Input: part model. Units: mm. Frame: model coordinates. A direction names the side the tool comes from. Round coordinates to 2 decimals unless told otherwise and drop trailing zeros. Use one line per item in the form item = value.
```python
from build123d import *

# Parameters (mm, degrees)
F1_DEPTH = 7.62


with BuildPart() as f1:
    # F0 (on Right) → F1 (new body)
    with BuildSketch(Plane.YZ):
        with BuildLine():
            Line((-83.8999077678, 0), (-76.0438218713, 0))
            Line((-76.0438218713, 0), (-68.3361637849, 0))
            Line((-68.3361637849, 0), (-65.6663442796, 0))
            Line((-65.6663442796, 0), (-59.0906857838, 0))
            Line((-59.0906857838, 0), (-56.6208846061, 0))
            Line((-56.6208846061, 0), (-50.1111261547, 0))
            Line((-50.1111261547, 0), (-47.2127646201, 0))
            Line((-47.2127646201, 0), (-40.9584082663, 0))
            Line((-40.9584082663, 0), (-38.0600504577, 0))
            Line((-38.0600504577, 0), (-31.6531471908, 0))
            Line((-31.6531471908, 0), (-28.9073325694, 0))
            Line((-28.9073325694, 0), (-22.5004293025, 0))
            Line((-22.5004293025, 0), (-19.9071597308, 0))
            Line((-19.9071597308, 0), (-13.4495065357, 0))
            Line((-13.4495065357, 0), (-10.754442774, 0))
            Line((-10.754442774, 0), (-4.1949953884, 0))
            Line((-4.1949953884, 0), (-1.6017258168, 0))
            Line((-1.6017258168, 0), (4.8051769845, 0))
            Line((4.8051769845, 0), (7.3984456249, 0))
            Line((7.3984456249, 0), (13.8053493574, 0))
            Line((13.8053493574, 0), (16.7037080973, 0))
            Line((16.7037080973, 0), (23.1106095016, 0))
            Line((23.1106095016, 0), (25.7038809359, 0))
            Line((25.7038809359, 0), (32.1107842028, 0))
            Line((32.1107842028, 0), (34.5515049994, 0))
            Line((34.5515049994, 0), (40.958404541, 0))
            Line((40.958404541, 0), (43.7042228877, 0))
            Line((43.7042228877, 0), (50.1111261552, 0))
            Line((50.1111261552, 0), (52.7043938637, 0))
            Line((52.7043938637, 0), (59.263844043, 0))
            Line((59.263844043, 0), (61.8571154775, 0))
            Line((61.8571154775, 0), (72.8403702378, 0))
            Line((72.8403702378, 0), (77.7980908751, 0))
            add(Edge.make_bspline(
                [(2.4155534392, 71.935541455), (28.1982811761, 69.4119022605), (52.9981860256, 34.7059511303), (77.7980908751, 0)],
                knots=[0.5202204491, 0.5202204491, 0.5202204491, 0.5202204491, 1, 1, 1, 1], degree=3))
            add(Edge.make_bspline(
                [(2.4155534392, 71.935541455), (23.457256807, 69.5741418959), (44.3202320999, 38.0280369375), (65.1832073927, 6.4819319791)],
                knots=[0.5194057291, 0.5194057291, 0.5194057291, 0.5194057291, 1, 1, 1, 1], degree=3))
            Line((65.1832073927, 6.4819319791), (29.4485222548, 6.4819319791))
            Line((29.4485222548, 6.4819319791), (17.7436252383, 6.4819319791))
            Line((17.7436252383, 6.4819319791), (-2.5848655496, 6.4819319791))
            Line((-2.5848655496, 6.4819319791), (-22.7159410715, 6.4819319791))
            Line((-22.7159410715, 6.4819319791), (-46.667508781, 6.4819319791))
            Line((-46.667508781, 6.4819319791), (-66.2550926208, 6.4819319791))
            add(Edge.make_bspline(
                [(-66.2550926208, 6.4819319791), (-44.7386888592, 38.3814174671), (-23.2222850975, 70.2809029552), (-1.8906832982, 72.0038712376)],
                knots=[0, 0, 0, 0, 0.4866401258, 0.4866401258, 0.4866401258, 0.4866401258], degree=3))
            add(Edge.make_bspline(
                [(-1.8906832982, 72.0038712376), (-1.2602925513, 72.0547883357), (-0.6300631821, 72.0793517198), (2.66e-08, 72.0767825841)],
                knots=[0.4866401258, 0.4866401258, 0.4866401258, 0.4866401258, 0.5010212977, 0.5010212977, 0.5010212977, 0.5010212977], degree=3))
            add(Edge.make_bspline(
                [(-83.8999077678, 0), (-55.5586168349, 36.2935873023), (-27.217325902, 72.5871746046), (0, 72.0767825842)],
                knots=[0, 0, 0, 0, 0.505255101, 0.505255101, 0.505255101, 0.505255101], degree=3))
        make_face()
        Polygon((-68.3361637849, 0), (-76.0438218713, 0), (-83.8999077678, 0), (-87.4847173691, 0), (-87.4847173691, -8.0094942823), (82.7558115125, -8.0094942823), (82.7558115125, 0), (77.7980908751, 0), (72.8403702378, 0), (61.8571154775, 0), (59.263844043, 0), (52.7043938637, 0), (50.1111261552, 0), (43.7042228877, 0), (40.958404541, 0), (34.5515049994, 0), (32.1107842028, 0), (25.7038809359, 0), (23.1106095016, 0), (16.7037080973, 0), (13.8053493574, 0), (7.3984456249, 0), (4.8051769845, 0), (-1.6017258168, 0), (-4.1949953884, 0), (-10.754442774, 0), (-13.4495065357, 0), (-19.9071597308, 0), (-22.5004293025, 0), (-28.9073325694, 0), (-31.6531471908, 0), (-38.0600504577, 0), (-40.9584082663, 0), (-47.2127646201, 0), (-50.1111261547, 0), (-56.6208846061, 0), (-59.0906857838, 0), (-65.6663442796, 0), align=None)
        with BuildLine():
            add(Edge.make_bspline(
                [(0, 72.0767825842), (0.8061606012, 72.0616650837), (1.6113351386, 72.0142591471), (2.4155534392, 71.935541455)],
                knots=[0.505255101, 0.505255101, 0.505255101, 0.505255101, 0.5202204491, 0.5202204491, 0.5202204491, 0.5202204491], degree=3))
            add(Edge.make_bspline(
                [(-1.8906832982, 72.0038712376), (-1.2602925513, 72.0547883357), (-0.6300631821, 72.0793517198), (2.66e-08, 72.0767825841)],
                knots=[0.4866401258, 0.4866401258, 0.4866401258, 0.4866401258, 0.5010212977, 0.5010212977, 0.5010212977, 0.5010212977], degree=3))
            add(Edge.make_bspline(
                [(-66.2550926208, 6.4819319791), (-44.7386888592, 38.3814174671), (-23.2222850975, 70.2809029552), (-1.8906832982, 72.0038712376)],
                knots=[0, 0, 0, 0, 0.4866401258, 0.4866401258, 0.4866401258, 0.4866401258], degree=3))
            add(Edge.make_bspline(
                [(-66.2550926208, 6.4819319791), (-58.870002531, 15.6014280008), (-51.4849124411, 24.7209240225), (-44.1068523116, 32.8232360474)],
                knots=[0, 0, 0, 0, 0.1671216862, 0.1671216862, 0.1671216862, 0.1671216862], degree=3))
            add(Edge.make_bspline(
                [(-44.1068523116, 32.8232360474), (-42.3619029204, 34.7394747588), (-40.6173467479, 36.5988175914), (-38.8732767924, 38.3878083756)],
                knots=[0.1671216862, 0.1671216862, 0.1671216862, 0.1671216862, 0.2066468296, 0.2066468296, 0.2066468296, 0.2066468296], degree=3))
            add(Edge.make_bspline(
                [(-38.8732767924, 38.3878083756), (-34.7114395699, 42.6568392208), (-30.5523710257, 46.5252625196), (-26.3973348433, 49.8102324575)],
                knots=[0.2066468296, 0.2066468296, 0.2066468296, 0.2066468296, 0.3009648428, 0.3009648428, 0.3009648428, 0.3009648428], degree=3))
            add(Edge.make_bspline(
                [(-26.3973348433, 49.8102324575), (-22.8832827761, 52.5884406113), (-19.3721149148, 54.9493251989), (-15.8645956908, 56.7822785692)],
                knots=[0.3009648428, 0.3009648428, 0.3009648428, 0.3009648428, 0.3807327183, 0.3807327183, 0.3807327183, 0.3807327183], degree=3))
            add(Edge.make_bspline(
                [(-15.8645956908, 56.7822785692), (-11.3638797078, 59.1342549956), (-6.8691712251, 60.6169899499), (-2.3820852822, 60.9967989829)],
                knots=[0.3807327183, 0.3807327183, 0.3807327183, 0.3807327183, 0.4830878387, 0.4830878387, 0.4830878387, 0.4830878387], degree=3))
            add(Edge.make_bspline(
                [(-2.3820852822, 60.9967989829), (-1.5878150287, 61.0640299254), (2.3324808206, 61.2253407539), (6.2467363494, 60.5126612784), (9.3648919901, 59.4680160873)],
                knots=[0.4830878387, 0.4830878387, 0.4830878387, 0.4830878387, 0.5012059734, 0.5725407835, 0.5725407835, 0.5725407835, 0.5725407835], degree=3))
            add(Edge.make_bspline(
                [(9.3648919901, 59.4680160873), (28.0498000323, 53.2081940706), (46.6165037125, 29.8450630249), (65.1832073927, 6.4819319791)],
                knots=[0.5725407835, 0.5725407835, 0.5725407835, 0.5725407835, 1, 1, 1, 1], degree=3))
            add(Edge.make_bspline(
                [(2.4155534392, 71.935541455), (23.457256807, 69.5741418959), (44.3202320999, 38.0280369375), (65.1832073927, 6.4819319791)],
                knots=[0.5194057291, 0.5194057291, 0.5194057291, 0.5194057291, 1, 1, 1, 1], degree=3))
        make_face()
        with BuildLine():
            Line((-37.4757476613, 19.9564792332), (-66.2550926208, 6.4819319791))
            Line((-66.2550926208, 6.4819319791), (-46.667508781, 6.4819319791))
            Line((-46.667508781, 6.4819319791), (-26.5364367513, 19.9564792332))
            Line((-26.5364367513, 19.9564792332), (-38.8732767924, 38.3878083756))
            add(Edge.make_bspline(
                [(-44.1068523116, 32.8232360474), (-42.3619029204, 34.7394747588), (-40.6173467479, 36.5988175914), (-38.8732767924, 38.3878083756)],
                knots=[0.1671216862, 0.1671216862, 0.1671216862, 0.1671216862, 0.2066468296, 0.2066468296, 0.2066468296, 0.2066468296], degree=3))
            Line((-44.1068523116, 32.8232360474), (-37.4757476613, 19.9564792332))
        make_face()
        with BuildLine():
            Line((17.7436252383, 6.4819319791), (29.4485222548, 6.4819319791))
            Line((29.4485222548, 6.4819319791), (43.261088431, 19.9564792332))
            Line((43.261088431, 19.9564792332), (9.3648919901, 59.4680160873))
            add(Edge.make_bspline(
                [(-2.3820852822, 60.9967989829), (-1.5878150287, 61.0640299254), (2.3324808206, 61.2253407539), (6.2467363494, 60.5126612784), (9.3648919901, 59.4680160873)],
                knots=[0.4830878387, 0.4830878387, 0.4830878387, 0.4830878387, 0.5012059734, 0.5725407835, 0.5725407835, 0.5725407835, 0.5725407835], degree=3))
            Line((-2.3820852822, 60.9967989829), (30.9179425241, 19.9564792332))
            Line((30.9179425241, 19.9564792332), (17.7436252383, 6.4819319791))
        make_face()
        with BuildLine():
            Line((0, 19.9564792332), (-22.7159410715, 6.4819319791))
            Line((-22.7159410715, 6.4819319791), (-2.5848655496, 6.4819319791))
            Line((-2.5848655496, 6.4819319791), (14.0195973219, 19.9564792332))
            Line((14.0195973219, 19.9564792332), (-15.8645956908, 56.7822785692))
            add(Edge.make_bspline(
                [(-26.3973348433, 49.8102324575), (-22.8832827761, 52.5884406113), (-19.3721149148, 54.9493251989), (-15.8645956908, 56.7822785692)],
                knots=[0.3009648428, 0.3009648428, 0.3009648428, 0.3009648428, 0.3807327183, 0.3807327183, 0.3807327183, 0.3807327183], degree=3))
            Line((-26.3973348433, 49.8102324575), (0, 19.9564792332))
        make_face()
    extrude(amount=F1_DEPTH)


solid = f1.part
```
(1) Cut plane A-A on x = 3.75. Count the separate pieces of the cut face and the enclosed holes in it, then the cut area to 3 significant figures.
Derived:
separate_pieces = 1
enclosed_holes = 4
area = 5,890 mm^2
(2) Draft query along Y for faces 1 (the face through (3.757, 26.55, 39.436)), 2 (the face through (3.76, -0.71, 38.11)), 3 (the face through (4, -87.485, -4)), 4 (the face through (4, -4, -8.009)). Return one class per face: released by +Y, released by -Y, zero draft, split by the parting line, or undercut.
Derived:
face_1 = undercut
face_2 = undercut
face_3 = released by -Y
face_4 = zero draft
(3) Access query for faces 5 (the face through (4, -86, 0)), 6 (the face through (3.757, -51.664, 13.314)), 7 (the face through (4, 80, 0)), 8 (the face through (7.62, -4, 15)), 9 (the face through (0, -4, 15)). Directions: +Z, -Z, +X, -X, +Y, -Y. A direction counts if a zero-diameter tool reaches every point of the face in a straight line with its end or side. Return the directions, or none.
Derived:
face_5 = +Z, +X, -X, -Y
face_6 = +X, -X
face_7 = +Z, +X, -X, +Y
face_8 = +Z, -Z, +X, +Y, -Y
face_9 = +Z, -Z, -X, +Y, -Y
(4) First-contact query: pin 1 Ø4 at (x, y) = (5.5, 81) entering from +Z; pin 2 Ø1 at (x, z) = (3.5, 8) entering from +Y; pin 3 Ø4 at (x, z) = (3, 51) entering from +Y. Flat tips, straight axial feed; report the tip coordinate or a pass-through.
Derived:
pin_1 = 0
pin_2 = 72.43
pin_3 = 39.56
(5) Material intervals for L1, parallel to Z at x = 6.5, y = -5.5; L2, parallel to Y at x = 4.5, z = 58; L3, parallel to Y at x = 1, z = 44, sorted ascending.
Derived:
L1 = -8.01 to 16.69, 26.18 to 44.01, 60.56 to 71.69
L2 = -32.37 to -13.36, 0.05 to 10.62, 13.09 to 30.16
L3 = -47.33 to -33.14, -21.26 to -5.49, 11.41 to 22.63, 32.64 to 44.16
